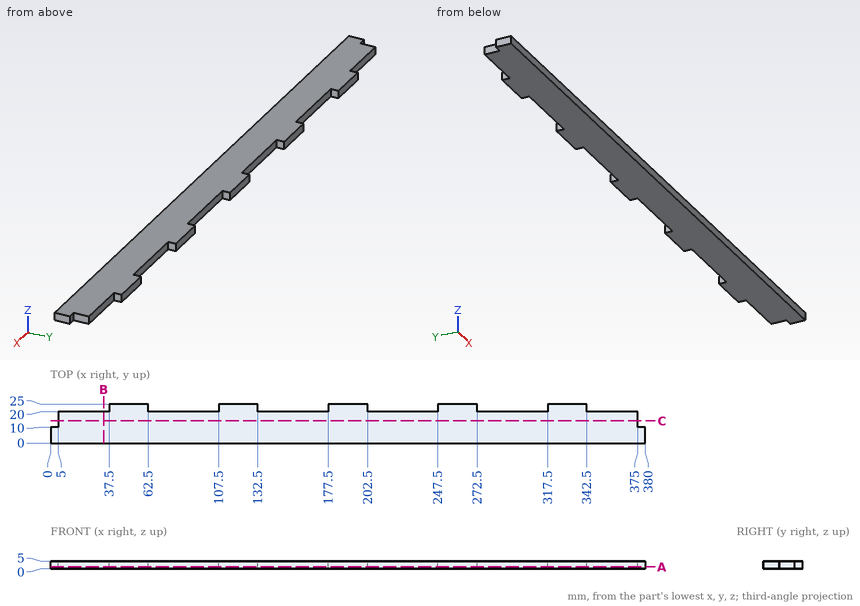
Job drawing, mm, ordinate dimensions from the low corner. One solid piece. Coordinates: 2 decimals unless noted, no trailing zeros. Order: outer loops, then holes, each group sorted by start corner. A loop starts at its lowest first (then second) coordinate and runs counter-clockwise, first axis right, second up. Notation, with made-up numbers: M -37,-12.75 L 8,-12.75 A10 cw 8,-5.75 Z; hole C 79,-36.5 d4. An arc over 180 degrees is marked long. Answer as CSV lines item,"result".
(1) Band-saw the part on A-A, the plane z = 1.3. List the corners of the cut face in (x, y), then the cut area to 4 significant figures.
Geometry says:
outline,"M 0,0 L 380,0 L 380,10 L 375,10 L 375,20 L 342.5,20 L 342.5,25 L 317.5,25 L 317.5,20 L 272.5,20 L 272.5,25 L 247.5,25 L 247.5,20 L 202.5,20 L 202.5,25 L 177.5,25 L 177.5,20 L 132.5,20 L 132.5,25 L 107.5,25 L 107.5,20 L 62.5,20 L 62.5,25 L 37.5,25 L 37.5,20 L 5,20 L 5,10 L 0,10 Z"
area,"8,125 mm2"
(2) Band-saw the part on C-C, the plane y = 14.25. List the corners of the cut face in (x, z), then the cut area to 3 significant figures.
Geometry says:
outline,"M 5,0 L 375,0 L 375,5 L 5,5 Z"
area,"1,850 mm2"
(3) Wall check: line 1 along X through (y, z) = (22.75, 1.45); line 2 along Y through (x, z) = (217, 1.3); line 3 along X through (y, z) = (13.5, 0.6). Give the ranges that are in metal, low to high.
Geometry says:
line 1,"x = 37.5 to 62.5, 107.5 to 132.5, 177.5 to 202.5, 247.5 to 272.5, 317.5 to 342.5"
line 2,"y = 0 to 20"
line 3,"x = 5 to 375"
(4) Band-saw the part on B-B, the plane x = 34. List the corners of the cut face in (y, z).
Geometry says:
outline,"M 0,0 L 20,0 L 20,5 L 0,5 Z"
(5) Flat gauge pins, fed straight in: pin 1 (1.5 mm diameter, centred on x = 3, z = 3.5, fed in from +Y); pin 2 (2.5 mm diameter, centred on y = 14, z = 3.5, fed in from -X); pin 3 (1.5 mm diameter, centred on y = 22, z = 3, fed in from +X). Where does each tip first touch, or does it go through?
Geometry says:
pin 1,"stops at y = 10"
pin 2,"stops at x = 5"
pin 3,"stops at x = 342.5"
